The listing builds one solid part. Answer for the finished solid, in the listing's coordinates (mm). A direction names the side the tool comes from. Round coordinates to 2 decimals unless told otherwise and drop trailing zeros. Write each loop counter-clockwise with the first axis right and the second up, starting at its lowest first coordinate (ties: lowest second). Pieces come first, ordered by that corner, then holes. Notation, with made-up numbers: (10, -28.75) - (20, -28.75) arc R27 ccw to (20, 3.25) - close; hole circle Ø8 at (56, 54). An arc over 180 degrees is marked (long way). Answer in a Markdown table with one row per item.
from build123d import *

# Parameters (mm, degrees)
F1_W     = 165.1
F1_H     = 154.2292288029
F2_DEPTH = 165.1
F3_R     = 27.6489440809
F4_DEPTH = 247.396
F5_W     = 92.6118567586
F5_H     = 56.6696990281
F6_DEPTH = 25.4


# Not quite as in the source:
# - a variable given as a bare number and used for a length is read in inches; the dataset says mm whatever the document's units were


with BuildPart() as f2:
    # F1 (on Top) → F2 (new body)
    with BuildSketch(Plane.XY):
        Rectangle(F1_W, F1_H)
    extrude(amount=F2_DEPTH)

    # F3 (on face) → F4 (cut)
    with BuildSketch(Plane.YZ.offset(82.55)):
        with Locations((-12.199181132, 81.3155397773)):
            Circle(F3_R)
    extrude(amount=-F4_DEPTH, mode=Mode.SUBTRACT)

    # F5 (on face) → F6 (cut)
    with BuildSketch(Plane.XY.offset(165.1)):
        with Locations((28.7659913301, -20.8643507212)):
            Rectangle(F5_W, F5_H)
    extrude(amount=-F6_DEPTH, mode=Mode.SUBTRACT)


solid = f2.part
(1) A flat-ended cylindrical pin translates along its axis: pin 1 (12 mm diameter, centred on x = 34, y = -5, fed in from +Z). Find the tip coordinate at first contact, or state that the pin passes through.
Checked values:
| item | result |
|---|---|
| pin 1 | stops at z = 139.7 |
(2) Section D-D (x = 24) is taken. Give the vertices of the cut face in (y, z), and give its area (3 significant figures).
Checked values:
| item | result |
|---|---|
| outline | (-77.11, 0) - (77.11, 0) - (77.11, 165.1) - (7.47, 165.1) - (7.47, 139.7) - (-49.2, 139.7) - (-49.2, 165.1) - (-77.11, 165.1) - close; hole circle Ø55.3 at (-12.2, 81.32) |
| area | 21,600 mm2 |
(3) For faces 5 (the flat face through (-1, -77.115, 81)), 6 (the flat face through (28, 7.47, 153)), determine the directions among +Z, -Z, +X, -X, +Y, -Y from which every point of the face is accessible in a straight line to the end or side of a thin tool.
Checked values:
| item | result |
|---|---|
| face 5 | +Z, -Z, +X, -X, -Y |
| face 6 | +Z |
(4) Section B-B (y = 13) is taken. Give the vertices of the cut face in (x, z), and give its area (3 significant figures).
Checked values:
| item | result |
|---|---|
| outline | (-82.55, 0) - (82.55, 0) - (82.55, 69.94) - (-82.55, 69.94) - close; (-82.55, 92.69) - (82.55, 92.69) - (82.55, 165.1) - (-82.55, 165.1) - close |
| area | 23,500 mm2 |
(5) For a pull along X with two mould halves and no side action, classify faces 1 (the flat face through (-1, 77.115, 81)), 2 (the flat face through (75.072, -21, 153)), 3 (the flat face through (-82.55, 16, 81)), 4 (the flat face through (82.55, 16, 81)) as pulls with the +X half, pulls with the -X half, needs draft (parallel to the pull), parting line crosses it, or undercut.
Checked values:
| item | result |
|---|---|
| face 1 | needs draft |
| face 2 | undercut |
| face 3 | pulls with the -X half |
| face 4 | pulls with the +X half |
(6) Section A-A (z = 144) is taken. Give the vertices of the cut face in (x, y).
Checked values:
| item | result |
|---|---|
| outline | (-82.55, -77.11) - (82.55, -77.11) - (82.55, 77.11) - (-82.55, 77.11) - close; hole (-17.54, -49.2) - (75.07, -49.2) - (75.07, 7.47) - (-17.54, 7.47) - close |
(7) Find the intervals of material crossed by line 1 (Z direction, x = -37.5, y = -12); line 2 (Y direction, x = 42, z = 141); line 3 (X direction, y = -25.5, z = 152), in increasing order.
Checked values:
| item | result |
|---|---|
| line 1 | z = 0 to 53.67, 108.96 to 165.1 |
| line 2 | y = -77.11 to -49.2, 7.47 to 77.11 |
| line 3 | x = -82.55 to -17.54, 75.07 to 82.55 |
(8) Section C-C (z = 63) is taken. Give the vertices of the cut face in (x, y), and give its area (3 significant figures).
Checked values:
| item | result |
|---|---|
| outline | (-82.55, -77.11) - (82.55, -77.11) - (82.55, -32.91) - (-82.55, -32.91) - close; (-82.55, 8.51) - (82.55, 8.51) - (82.55, 77.11) - (-82.55, 77.11) - close |
| area | 18,600 mm2 |
